Design review of the part built by this model. Coordinates are the model's own, in mm. Face numbers are marked on the shaded views. A direction names the side the tool comes from. Round coordinates to 2 decimals unless told otherwise and drop trailing zeros. Loops run counter-clockwise (first coordinate to the right, second up) from the corner with the lowest first, then second, coordinate; pieces in that order, holes last. Notation, with made-up numbers: M -30.75,57.25 L -11.75,57.25 A17 ccw -11.75,69.25 Z; hole C 30.5,-29 d3. An arc over 180 degrees is marked long. Use a Markdown table: item, result.
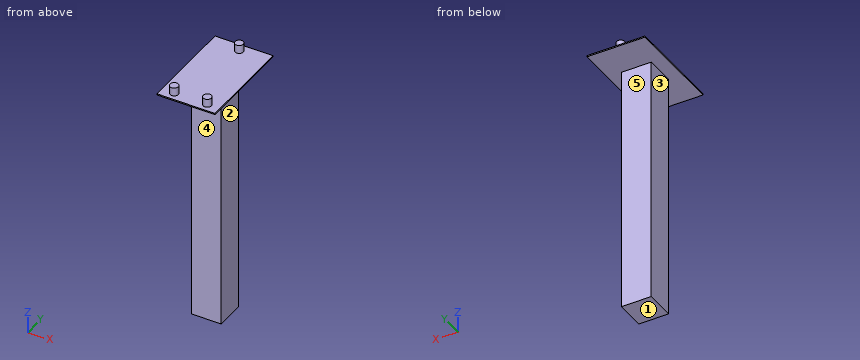
from build123d import *

# Parameters (mm, degrees)
SKETCH1_W           = 36
SKETCH1_H           = 36
BOSS_EXTRUDE1_DEPTH = 300
SKETCH2_W           = 70
SKETCH2_H           = 120
BOSS_EXTRUDE2_DEPTH = 1.5
SKETCH3_R           = 5
BOSS_EXTRUDE3_DEPTH = 10


with BuildPart() as part:
    # Sketch1 → Boss-Extrude1 (new body)
    with BuildSketch(Plane.XY):
        Rectangle(SKETCH1_W, SKETCH1_H)
    extrude(amount=BOSS_EXTRUDE1_DEPTH)

    # Sketch2 → Boss-Extrude2 (add)
    with BuildSketch(Plane.XY.offset(300)):
        Rectangle(SKETCH2_W, SKETCH2_H)
    extrude(amount=BOSS_EXTRUDE2_DEPTH)

    # Sketch3 → Boss-Extrude3 (add)
    with BuildSketch(Plane.XY.offset(301.5)):
        with Locations((0, 50)):
            Circle(SKETCH3_R)
        with Locations((-20, -50)):
            Circle(SKETCH3_R)
        with Locations((20, -50)):
            Circle(SKETCH3_R)
    extrude(amount=BOSS_EXTRUDE3_DEPTH)


solid = part.part
1. Take a section at A-A on y = -50. Give the boundary of the cut face in (x, z), and give its area (3 significant figures).
Check values:
| item | result |
|---|---|
| outline | M -35,300 L 35,300 L 35,301.5 L 25,301.5 L 25,311.5 L 15,311.5 L 15,301.5 L -15,301.5 L -15,311.5 L -25,311.5 L -25,301.5 L -35,301.5 Z |
| area | 305 mm² |
2. Insertion check: pin 1 (3 mm diameter, centred on x = 8.5, y = -30, fed in from +Z); pin 2 (12 mm diameter, centred on x = -13, z = 120.5, fed in from -Y); pin 3 (18 mm diameter, centred on y = -1, z = 125.5, fed in from -X). Each pin has a flat end and moves straight along its axis. Give the tip position at first contact, or say it passes through.
Check values:
| item | result |
|---|---|
| pin 1 | stops at z = 301.5 |
| pin 2 | stops at y = -18 |
| pin 3 | stops at x = -18 |
3. Take a section at D-D on z = 198.5. Give the boundary of the cut face in (x, y).
Check values:
| item | result |
|---|---|
| outline | M -18,-18 L 18,-18 L 18,18 L -18,18 Z |
4. Wall thickness on line 1 along X through (y, z) = (6, 214.5); line 2 along Z through (x, y) = (16, 49.5): over which ranges is each line inside the solid? List them lowest first. Write a range as from..to.
Check values:
| item | result |
|---|---|
| line 1 | x = -18..18 |
| line 2 | z = 300..301.5 |
5. Machinability: for the marked faces 1, 2, 3, 4 and 5, which of the approach directions +Z, -Z, +X, -X, +Y, -Y give a long, thin tool a straight path to every point of the face, cutting with its end or side? Answer none if there is none.
Check values:
| item | result |
|---|---|
| face 1 | -Z, +X, -X, +Y, -Y |
| face 2 | -Z, +X, +Y, -Y |
| face 3 | -Z, -X, +Y, -Y |
| face 4 | -Z, +X, -X, -Y |
| face 5 | -Z, +X, -X, +Y |
6. Take a section at C-C on y = 1. Give the boundary of the cut face in (x, z).
Check values:
| item | result |
|---|---|
| outline | M -35,300 L -18,300 L -18,0 L 18,0 L 18,300 L 35,300 L 35,301.5 L -35,301.5 Z |
7. Take a section at B-B on x = 0. Give the boundary of the cut face in (y, z), and give its area (3 significant figures).
Check values:
| item | result |
|---|---|
| outline | M -60,300 L -18,300 L -18,0 L 18,0 L 18,300 L 60,300 L 60,301.5 L 55,301.5 L 55,311.5 L 45,311.5 L 45,301.5 L -60,301.5 Z |
| area | 11,100 mm² |
